from build123d import *

# Parameters (mm, degrees)
F0_W     = 88.9
F0_H     = 88.9
F1_DEPTH = 92.075
F2_R     = 6.35
F3_DEPTH = 50.8
F4_R     = 6.35
F5_DEPTH = 50.8


with BuildPart() as f1:
    # F0 (on Top) → F1 (new body, symmetric)
    with BuildSketch(Plane.XY):
        Rectangle(F0_W, F0_H)
    extrude(amount=F1_DEPTH, both=True)

    # F2 (on Front) → F3 (cut, symmetric)
    with BuildSketch(Plane.XZ):
        with Locations((0, 76.2)):
            Circle(F2_R)
        with Locations((0, -50.8)):
            Circle(F2_R)
    extrude(amount=F3_DEPTH, both=True, mode=Mode.SUBTRACT)

    # F4 (on Right) → F5 (cut, symmetric)
    with BuildSketch(Plane.YZ):
        with Locations((0, 50.8)):
            Circle(F4_R)
        with Locations((0, -76.2)):
            Circle(F4_R)
    extrude(amount=F5_DEPTH, both=True, mode=Mode.SUBTRACT)


solid = f1.part
Verification items for the finished model (mm, model axes). Give positions to 0.01 mm unless a question says otherwise; leave off trailing zeros. Write each loop counter-clockwise with the first axis right and the second up, starting at its lowest first coordinate (ties: lowest second). Pieces come first, ordered by that corner, then holes.
(1) Cross-section at B-B (y = 0). Enter the section's corners in (x, z) (3 decimals).
(2) Cross-section at A-A (x = 0). Enter the section's corners in (y, z) (3 decimals).
(3) Cross-section at C-C (z = -76.2). Enter the section's corners in (x, y).
(4) Gauge pin test, flat ends, axial feed: pin 1 (20.5 mm diameter, centred on x = 0, z = 76.2, fed in from +Y); pin 2 (7.5 mm diameter, centred on x = 0, z = -50.8, fed in from -Y). Record the tip position at first contact, or that the pin passes through.
(5) Mould release check, pull along Z, two halves, no side actions. Record for faces 1 (the face through (-1, -44.45, 1)), 2 (the face through (-1, 1, 92.075)), 3 (the face through (0.6, -0.8, 57.1)): +Z half, -Z half, draft (parallel to the pull), parting line (faces both ways), or undercut.
(6) Material ranges on line 1 (Z direction, x = 0, y = 18) (3 decimals); line 2 (X direction, y = -24, z = 76.2), recorded low to high.
(7) Cross-section at D-D (x = 10). Enter the section's corners in (y, z) (3 decimals).
Worked out:
1. outline: (-44.45, -92.075) - (44.45, -92.075) - (44.45, -82.55) - (-44.45, -82.55) - close; (-44.45, -69.85) - (44.45, -69.85) - (44.45, 44.45) - (-44.45, 44.45) - close; (-44.45, 57.15) - (44.45, 57.15) - (44.45, 92.075) - (-44.45, 92.075) - close; hole circle Ø12.7 at (0, -50.8); hole circle Ø12.7 at (0, 76.2)
2. outline: (-44.45, -92.075) - (44.45, -92.075) - (44.45, -57.15) - (-44.45, -57.15) - close; (-44.45, -44.45) - (44.45, -44.45) - (44.45, 69.85) - (-44.45, 69.85) - close; (-44.45, 82.55) - (44.45, 82.55) - (44.45, 92.075) - (-44.45, 92.075) - close; hole circle Ø12.7 at (0, -76.2); hole circle Ø12.7 at (0, 50.8)
3. outline: (-44.45, -44.45) - (44.45, -44.45) - (44.45, -6.35) - (-44.45, -6.35) - close; (-44.45, 6.35) - (44.45, 6.35) - (44.45, 44.45) - (-44.45, 44.45) - close
4. pin 1: stops at y = 44.45
4. pin 2: passes through
5. face 1: draft
5. face 2: +Z half
5. face 3: undercut
6. line 1: z = -92.075 to -57.15, -44.45 to 69.85, 82.55 to 92.075
6. line 2: x = -44.45 to -6.35, 6.35 to 44.45
7. outline: (-44.45, -92.075) - (44.45, -92.075) - (44.45, 92.075) - (-44.45, 92.075) - close; hole circle Ø12.7 at (0, -76.2); hole circle Ø12.7 at (0, 50.8)
